Work out the finished part from the listing and answer in its coordinate system (mm). A direction names the side the tool comes from. Coordinates: 2 decimals unless noted, no trailing zeros. Write each loop counter-clockwise with the first axis right and the second up, starting at its lowest first coordinate (ties: lowest second). Pieces come first, ordered by that corner, then holes. Notation, with made-up numbers: (-27.75, 51) - (18.25, 51) arc R28 ccw to (18.25, 69) - close; hole circle Ø9 at (-1, 69). An arc over 180 degrees is marked (long way). One line per item, written item: value.
```python
from build123d import *

# Parameters (mm, degrees)
BOSS_EXTRUDE1_DEPTH = 491.49
SKETCH2_R           = 38.1
BOSS_EXTRUDE2_DEPTH = 38.1
SKETCH3_R           = 38.1
BOSS_EXTRUDE3_DEPTH = 38.1


with BuildPart() as part:
    # Sketch1 → Boss-Extrude1 (new body)
    with BuildSketch(Plane(origin=(0, 0, 0), x_dir=(0, 0, -1), z_dir=(1, 0, 0))):
        with BuildLine():
            Line((27.94, 6.35), (27.94, -6.35))
            Line((27.94, -6.35), (37.567106623, -6.35))
            ThreePointArc((37.567106623, -6.35), (37.966542918, -3.186160517), (38.1, 0))
            ThreePointArc((38.1, 0), (37.966542918, 3.186160517), (37.567106623, 6.35))
            Line((37.567106623, 6.35), (27.94, 6.35))
        make_face()
        with BuildLine():
            Line((37.567106623, -6.35), (27.94, -6.35))
            Line((27.94, -6.35), (27.94, 6.35))
            Line((27.94, 6.35), (37.567106623, 6.35))
            ThreePointArc((37.567106623, 6.35), (-38.1, 0), (37.567106623, -6.35))
        make_face()
        with BuildLine():
            ThreePointArc((38.1, 0), (37.966542918, -3.186160517), (37.567106623, -6.35))
            Line((37.567106623, -6.35), (48.26, -6.35))
            Line((48.26, -6.35), (48.26, 6.35))
            Line((48.26, 6.35), (37.567106623, 6.35))
            ThreePointArc((37.567106623, 6.35), (37.966542918, 3.186160517), (38.1, 0))
        make_face()
    extrude(amount=-BOSS_EXTRUDE1_DEPTH)

    # Sketch2 → Boss-Extrude2 (add)
    with BuildSketch(Plane(origin=(0, 0, 0), x_dir=(0, 0, -1), z_dir=(1, 0, 0))):
        Circle(SKETCH2_R)
    extrude(amount=BOSS_EXTRUDE2_DEPTH)

    # Sketch3 → Boss-Extrude3 (add)
    with BuildSketch(Plane.ZY.offset(491.49)):
        Circle(SKETCH3_R)
    extrude(amount=BOSS_EXTRUDE3_DEPTH)


solid = part.part
```
Item 1: Section B-B, the plane x = -414 is taken. Determine the outline of the cut face in (y, z).
Evaluation:
outline: (-6.35, -48.26) - (6.35, -48.26) - (6.35, -37.57) arc R38.1 ccw (long way) to (-6.35, -37.57) - close
Item 2: Which of the six approach directions +Z, -Z, +X, -X, +Y, -Y give full straight-line access (tool end or side, diameter ignored) to faces 1 (the face through (-242, 0, -48.26)), 2 (the face through (-242, 6.35, -43)), 3 (the face through (-242, -6.35, -43))?
Evaluation:
face 1: -Z, +X, -X, +Y, -Y
face 2: -Z, +X, -X, +Y
face 3: -Z, +X, -X, -Y
Item 3: Given pin 1 (12 mm diameter, centred on x = -283, z = -40.5, fed in from +Y); pin 2 (12 mm diameter, centred on x = -230, z = -23.5, fed in from -Y); pin 3 (1.5 mm diameter, centred on x = -212, y = -8.5, fed in from +Z), each flat-ended and moving along its own axis, determine where each tip first touches the part or whether it passes through.
Evaluation:
pin 1: stops at y = 16.17
pin 2: stops at y = -33.84
pin 3: stops at z = 37.3
Item 4: Section C-C, the plane z = -15 is taken. Determine the outline of the cut face in (x, y).
Evaluation:
outline: (-529.59, -35.02) - (38.1, -35.02) - (38.1, 35.02) - (-529.59, 35.02) - close
Item 5: Section A-A, the plane y = 0 is taken. Determine the outline of the cut face in (x, z), then the cut area to 3 significant figures.
Evaluation:
outline: (-529.59, -38.1) - (-491.49, -38.1) - (-491.49, -48.26) - (0, -48.26) - (0, -38.1) - (38.1, -38.1) - (38.1, 38.1) - (-529.59, 38.1) - close
area: 48,300 mm2
Item 6: Consider probe 1 along X at (y, z) = (4, -39.5); probe 2 along Z at (x, y) = (2.5, -1); probe 3 along Y at (x, z) = (-101.5, -38.5). Determine where each line is inside the solid, lowest interval first.
Evaluation:
probe 1: x = -491.49 to 0
probe 2: z = -38.09 to 38.09
probe 3: y = -6.35 to 6.35
